Read the model definition and answer for the solid it produces. Units are mm, in the model's axes. A direction names the side the tool comes from. Give positions to 0.01 mm unless a question says otherwise; leave off trailing zeros. Loops run counter-clockwise (first coordinate to the right, second up) from the corner with the lowest first, then second, coordinate; pieces in that order, holes last. Notation, with made-up numbers: (-39.75, -10) -> (-10.75, -10) arc R21 ccw to (-10.75, 17) -> close; hole circle Ø2 at (-34.5, 89.25). An arc over 180 degrees is marked (long way). Return JSON: item names as keys, results as strings. Group by question number.
Autodesk Inventor part; units mm, degrees
ref_plane "YZ Plane" through (0, 0, 0) normal (1, 0, 0) x (0, 1, 0)
ref_plane "XZ Plane" through (0, 0, 0) normal (0, 1, 0) x (-1, 0, 0)
ref_plane "XY Plane" through (0, 0, 0) normal (0, 0, 1) x (1, 0, 0)
sketch "Sketch1" plane through (0, 0, 0) normal (0, 1, 0) x (-1, 0, 0)
  line L0 (0, 0) -> (0, 69.2)
  line L1 (46.8, 69.2) -> (63.2, 69.2)
  line L2 (0, 69.2) -> (46.8, 69.2) construction
  line L3 (63.2, 69.2) -> (63.2, 0)
  line L4 (63.2, 0) -> (55, 0)
  line L5 (55, 0) -> (55, 61)
  line L6 (55, 0) -> (0, 0) construction
  line L7 (-281, 281) -> (-211.8, 281)
  line L8 (-211.8, 281) -> (-211.8, 234.2) construction
  line L9 (-281, 217.8) -> (-281, 226)
  line L10 (-281, 226) -> (-220, 226)
  line L11 (-281, 226) -> (-281, 281) construction
  line L12 (-211.8, 281) -> (0, 281) construction
  line L13 (0, 281) -> (0, 69.2) construction
  line L14 (46.8, 69.2) -> (46.8, 61)
  line L15 (46.8, 61) -> (55, 61)
  line L16 (-211.8, 234.2) -> (-220, 234.2)
  line L17 (-220, 234.2) -> (-220, 226)
  line L18 (-281, 217.8) -> (-211.8, 217.8)
  line L19 (-211.8, 234.2) -> (-211.8, 217.8)
  line L20 (-220, 234.2) -> (-220, 281) construction
  line L21 (46.8, 61) -> (0, 61) construction
  dimension "d0" = 110
  dimension "d1" = 8.2
  dimension "d2" = 61
  dimension "d4" = 93.6
  dimension "d6" = 110
  dimension "d7" = 93.6
  dimension "d10" = 8.2
  dimension "d11" = 8.2
  dimension "d12" = 61
  dimension "d14" = 220
  dimension "d15" = 220
  dimension "d16" = 8.2
revolve "Revolution1" add sketch "Sketch1" angle 360 about axis through (0, 0, 0) along (0, 0, 1) contours L1 L3 L4 L5 L15 L14
sketch "Sketch2" plane through (0, 0, 0) normal (0, 1, 0) x (-1, 0, 0)
  line L0 (0, 69.2) -> (0, 281) construction
  line L1 (0, 281) -> (-211.8, 281) construction
  arc A0 (0, 69.2) -> (-211.8, 281) centre (-211.8, 69.2) ccw
  line L2 (-63.2, 69.2) -> (63.2, 69.2)
  dimension "d8" = 211.8
  dimension "d9" = 211.8
sketch "Sketch3" plane through (0, 0, 69.2) normal (0, 0, 1) x (1, 0, 0)
  circle A0 centre (0, 0) radius 55
  circle A1 centre (0, 0) radius 55
  circle A2 centre (0, 0) radius 46.8
  circle A3 centre (0, 0) radius 46.8
  dimension "d13" = 110
sweep "Sweep1" add profiles "Sketch3" path "Sketch2" path curves A0
revolve "Revolution2" add sketch "Sketch1" angle 360 about axis through (281, 0, 281) along (-1, 0, 0) contours L9 L10 L17 L16 L19 L18
equation "\"d0\" = D1"
equation "\"d1\" = S"
equation "\"d2\" = T"
equation "\"d4\" = D1 - 2 * S"
equation "\"d6\" = D1"
equation "\"d7\" = D1 - 2 * S"
equation "\"d10\" = S"
equation "\"d11\" = S"
equation "\"d12\" = T"
equation "\"d14\" = Z"
equation "\"d15\" = Z"
equation "\"d16\" = S"
equation "\"d8\" = Z - S"
equation "\"d9\" = Z - S"
equation "\"d13\" = D1"
equation "\"D1\" = 110"
equation "\"T\" = 61"
equation "\"Z\" = 220"
equation "\"S\" = 8.2"
properties part number "DIN 8063 Колено 90 градусов, тип B 110" material "ПВХ, непластифицированный"
1. Which of the six approach directions +Z, -Z, +X, -X, +Y, -Y give full straight-line access (tool end or side, diameter ignored) to faces 4 (the cylindrical face through (10.145, -45.687, 65.043)), 5 (the cylindrical face through (245.92, 24.21, 222.62)), 6 (the flat face through (19, -52, 0)), 7 (the flat face through (281, -52, 300)), 8 (the flat face through (211.8, -52, 300))?
2. Flat-ended cylindrical pins translate along their axes: pin 1 Ø3 at (x, y) = (34.5, 39.5) entering from +Z; pin 2 Ø3 at (x, y) = (58.5, -18.5) entering from -Z; pin 3 Ø5 at (y, z) = (43, 140.5) entering from +X; pin 4 Ø4 at (y, z) = (-23, 52.5) entering from -X. Find the tip coordinate at first contact, or state that the pin passes through.
3. Determine the mould class of faces 1 (the flat face through (29, -37, 61)), 2 (the cylindrical face through (50.15, -38.46, 34.12)), 3 (the cylindrical face through (250.07, -16.52, 228.54)) for opening direction Z: pulls with the +Z half, pulls with the -Z half, needs draft (parallel to the pull), parting line crosses it, or undercut.
4. Section B-B on y = -22 is taken. Determine the outline of the cut face in (x, z).
5. Straight lines are drawn through the part: line 1 (Z direction, x = 234, y = 0); line 2 (Y direction, x = 255, z = 281); line 3 (Y direction, x = 0, z = 67). For each, find the intervals that lie inside material, in ascending order. Write a range as from..to.
6. Section A-A on y = 0 is taken. Determine the outline of the cut face in (x, z), then the cut area to 3 significant figures.
Completed:
{
 "1": {"face 4": "-Z", "face 5": "+X", "face 6": "-Z, +X, -X, +Y, -Y", "face 7": "+Z, -Z, +X, +Y, -Y", "face 8": "none"},
 "2": {"pin 1": "stops at z = 248.14", "pin 2": "stops at z = 0", "pin 3": "stops at x = 52.64", "pin 4": "stops at x = -59.61"},
 "3": {"face 1": "pulls with the -Z half", "face 2": "needs draft", "face 3": "undercut"},
 "4": {"outline": "(-59.25, 0) -> (-50.41, 0) -> (-50.41, 61) -> (-41.31, 61) -> (-41.31, 69.2) arc R253.11 cw to (211.8, 322.31) -> (220, 322.31) -> (220, 331.41) -> (281, 331.41) -> (281, 340.25) -> (211.8, 340.25) -> (211.8, 331.41) arc R262.21 ccw to (-50.41, 69.2) -> (-59.25, 69.2) -> close; (41.31, 61) -> (50.41, 61) -> (50.41, 0) -> (59.25, 0) -> (59.25, 69.2) -> (50.41, 69.2) arc R161.39 cw to (211.8, 230.59) -> (211.8, 221.75) -> (281, 221.75) -> (281, 230.59) -> (220, 230.59) -> (220, 239.69) -> (211.8, 239.69) arc R170.49 ccw to (41.31, 69.2) -> close"},
 "5": {"line 1": "z = 217.8..226, 336..344.2", "line 2": "y = -63.2..-55, 55..63.2", "line 3": "y = -63.2..-46.8, 46.8..63.2"},
 "6": {"outline": "(-63.2, 0) -> (-55, 0) -> (-55, 61) -> (-46.8, 61) -> (-46.8, 69.2) arc R258.6 cw to (211.8, 327.8) -> (220, 327.8) -> (220, 336) -> (281, 336) -> (281, 344.2) -> (211.8, 344.2) -> (211.8, 336) arc R266.8 ccw to (-55, 69.2) -> (-63.2, 69.2) -> close; (46.8, 61) -> (55, 61) -> (55, 0) -> (63.2, 0) -> (63.2, 69.2) -> (55, 69.2) arc R156.8 cw to (211.8, 226) -> (211.8, 217.8) -> (281, 217.8) -> (281, 226) -> (220, 226) -> (220, 234.2) -> (211.8, 234.2) arc R165 ccw to (46.8, 69.2) -> close", "area": "7,990 mm²"}
}
